Here's how the part is built. I have some questions about the finished solid (model axes, mm). A direction names the side the tool comes from. Coordinates: 2 decimals unless noted, no trailing zeros. Write each loop counter-clockwise with the first axis right and the second up, starting at its lowest first coordinate (ties: lowest second). Pieces come first, ordered by that corner, then holes.
(1) Imagine slicing it at C-C, the plane z = -25.4. List the corners of the cut face in (x, y) for me, plus the area to 3 significant figures.
(2) Please list where these lines run through material, in increasing order: probe 1 along Z at (x, y) = (0, 0.5); probe 2 along Z at (x, y) = (10, 29.5); probe 3 along X at (y, z) = (60.5, 49.5).
(3) Thinking about a two-plate mould opening in Z: for faces 1 (the flat face through (-1, 38, -63.5)), 2 (the flat face through (1, 38, 63.5)), 3 (the flat face through (-50.8, 38, 1)), 4 (the cylindrical face through (0.96, 0.52, 27.25)), which applies, released by +Z, released by -Z, zero draft, split by the parting line, or undercut?
(4) Which directions (+Z, -Z, +X, -X, +Y, -Y) give clear straight access to the entire face, cutting with the end or side of a thin tool? Please do faces 5 (the flat face through (1, 1.016, 1)), 6 (the flat face through (50.8, 38, -1)).
(5) For pin 1 Ø3 at (x, z) = (-9.5, 7.5) entering from -Y; pin 2 Ø4 at (x, z) = (13, -2.5) entering from +Y, each with a flat end and sliding along its axis, tell me the tip position at first contact or that it passes through.
(6) Imagine slicing it at A-A, the plane y = 7.5. List the corners of the cut face in (x, z) for me.
(7) Imagine slicing it at B-B, the plane x = 0. List the corners of the cut face in (y, z) for me.
Autodesk Inventor part; units mm, degrees
ref_plane "YZ Plane" through (0, 0, 0) normal (1, 0, 0) x (0, 1, 0)
ref_plane "XZ Plane" through (0, 0, 0) normal (0, 1, 0) x (-1, 0, 0)
ref_plane "XY Plane" through (0, 0, 0) normal (0, 0, 1) x (1, 0, 0)
sketch "Sketch1" plane through (0, 0, 0) normal (0, 1, 0) x (-1, 0, 0)
  line L0 (-50.8, 63.5) -> (50.8, 63.5)
  line L1 (50.8, 63.5) -> (50.8, -63.5)
  line L2 (50.8, -63.5) -> (-50.8, -63.5)
  line L3 (-50.8, -63.5) -> (-50.8, 63.5)
  line L4 (-50.8, 63.5) -> (50.8, -63.5) construction
  line L5 (50.8, 63.5) -> (-50.8, -63.5) construction
  point P0 (0, 0)
  dimension "d0" = 101.6
  dimension "d1" = 127
extrude "Extrusion1" add sketch "Sketch1" along normal blind 1.016
sketch "Sketch2" plane through (0, 1.016, 0) normal (0, 1, 0) x (1, 0, 0)
  line L0 (50.8, 63.5) -> (-50.8, 63.5)
  line L1 (50.8, -63.5) -> (-50.8, -63.5)
  line L2 (-50.8, -63.5) -> (-50.8, 63.5)
  line L3 (-50.8, 63.5) -> (50.8, 63.5)
  line L4 (50.8, 63.5) -> (50.8, -63.5)
  line L5 (50.8, -63.5) -> (-50.8, 63.5) construction
  line L6 (-50.8, -63.5) -> (50.8, 63.5) construction
  line L7 (50.292, -62.992) -> (-50.292, -62.992)
  line L8 (-50.292, -62.992) -> (-50.292, 62.992)
  line L9 (-50.292, 62.992) -> (50.292, 62.992)
  line L10 (50.292, 62.992) -> (50.292, -62.992)
  line L11 (50.292, -62.992) -> (-50.292, 62.992) construction
  line L12 (-50.292, -62.992) -> (50.292, 62.992) construction
  point P0 (0, 0)
  dimension "d4" = 100.584
  dimension "d5" = 125.984
extrude "Extrusion2" add sketch "Sketch2" along normal blind 76.2
sketch "Sketch3" plane through (0, 1.016, 0) normal (0, 1, 0) x (1, 0, 0)
  line L0 (0, 0) -> (0, -25.4)
  line L1 (0, -25.4) -> (0, 25.4)
  circle A0 centre (0, -25.4) radius 2.0828
  circle A1 centre (0, 25.4) radius 2.0828
  dimension "d8" = 25.4
  dimension "d9" = 50.8
  dimension "d10" = 4.1656
  dimension "d11" = 4.1656
extrude "Extrusion3" cut sketch "Sketch3" against normal through all
properties part number "563-AU1028MG-5x4-Enclosure"
Recorded:
1. outline: (-50.8, 0) - (-2.08, 0) - (-2.08, 1.02) - (-50.29, 1.02) - (-50.29, 77.22) - (-50.8, 77.22) - close; (2.08, 0) - (50.8, 0) - (50.8, 77.22) - (50.29, 77.22) - (50.29, 1.02) - (2.08, 1.02) - close
1. area: 176 mm2
2. probe 1: z = -63.5 to -27.48, -23.32 to 23.32, 27.48 to 63.5
2. probe 2: z = -63.5 to -62.99, 62.99 to 63.5
2. probe 3: x = -50.8 to -50.29, 50.29 to 50.8
3. face 1: released by -Z
3. face 2: released by +Z
3. face 3: zero draft
3. face 4: undercut
4. face 5: +Y
4. face 6: +Z, -Z, +X, +Y, -Y
5. pin 1: stops at y = 0
5. pin 2: stops at y = 1.02
6. outline: (-50.8, -63.5) - (50.8, -63.5) - (50.8, 63.5) - (-50.8, 63.5) - close; hole (-50.29, -62.99) - (50.29, -62.99) - (50.29, 62.99) - (-50.29, 62.99) - close
7. outline: (0, -63.5) - (77.22, -63.5) - (77.22, -62.99) - (1.02, -62.99) - (1.02, -27.48) - (0, -27.48) - close; (0, -23.32) - (1.02, -23.32) - (1.02, 23.32) - (0, 23.32) - close; (0, 27.48) - (1.02, 27.48) - (1.02, 62.99) - (77.22, 62.99) - (77.22, 63.5) - (0, 63.5) - close
